from build123d import *

# Parameters (mm, degrees)
BOSS_EXTRUDE1_DEPTH = 4
SKETCH2_W           = 30
SKETCH2_H           = 22
BOSS_EXTRUDE2_DEPTH = 4
SKETCH3_W           = 30
SKETCH3_H           = 4
BOSS_EXTRUDE3_DEPTH = 18
CUT_EXTRUDE1_REACH  = 6
SKETCH4_R           = 2.25
CUT_EXTRUDE2_REACH  = 6
SKETCH5_W           = 12
SKETCH5_H           = 18


with BuildPart() as part:
    # Sketch1 → Boss-Extrude1 (new body)
    with BuildSketch(Plane(origin=(0, 0, 0), x_dir=(1, 0, 0), z_dir=(0, 1, 0))):
        with BuildLine():
            Line((-15, -14.5), (-9.788986692, -14.5))
            ThreePointArc((-9.788986692, -14.5), (-9, -10.35), (-8.211013308, -14.5))
            Line((-8.211013308, -14.5), (8.211013308, -14.5))
            ThreePointArc((8.211013308, -14.5), (9, -10.35), (9.788986692, -14.5))
            Line((9.788986692, -14.5), (15, -14.5))
            Line((15, -14.5), (15, 14.5))
            Line((15, 14.5), (-15, 14.5))
            Line((-15, 14.5), (-15, -14.5))
        make_face()
    extrude(amount=BOSS_EXTRUDE1_DEPTH)

    # Sketch2 → Boss-Extrude2 (add)
    with BuildSketch(Plane.XZ):
        with Locations((0, -3.5)):
            Rectangle(SKETCH2_W, SKETCH2_H)
    extrude(amount=BOSS_EXTRUDE2_DEPTH)

    # Sketch3 → Boss-Extrude3 (add)
    with BuildSketch(Plane(origin=(0, 0, -14.5), x_dir=(-1, 0, 0), z_dir=(0, 0, -1))):
        with Locations((0, 2)):
            Rectangle(SKETCH3_W, SKETCH3_H)
    extrude(amount=BOSS_EXTRUDE3_DEPTH)

    # Sketch4 → Cut-Extrude1 (cut, up to next)
    with BuildSketch(Plane(origin=(0, 0, 0), x_dir=(-1, 0, 0), z_dir=(0, 1, 0)), mode=Mode.PRIVATE) as cut_extrude1_sk1:
        with Locations((2, -27)):
            Circle(SKETCH4_R)
    cut_extrude1_tool1 = extrude(cut_extrude1_sk1.sketch, amount=CUT_EXTRUDE1_REACH, mode=Mode.PRIVATE) & part.part
    add(cut_extrude1_tool1.solids().sort_by_distance((-2, 0, -27))[0], mode=Mode.SUBTRACT)
    # Sketch4 → Cut-Extrude1 (cut, up to next)
    with BuildSketch(Plane(origin=(0, 0, 0), x_dir=(-1, 0, 0), z_dir=(0, 1, 0)), mode=Mode.PRIVATE) as cut_extrude1_sk2:
        with Locations((10, -23.5)):
            Circle(SKETCH4_R)
    cut_extrude1_tool2 = extrude(cut_extrude1_sk2.sketch, amount=CUT_EXTRUDE1_REACH, mode=Mode.PRIVATE) & part.part
    add(cut_extrude1_tool2.solids().sort_by_distance((-10, 0, -23.5))[0], mode=Mode.SUBTRACT)
    # Sketch4 → Cut-Extrude1 (cut, up to next)
    with BuildSketch(Plane(origin=(0, 0, 0), x_dir=(-1, 0, 0), z_dir=(0, 1, 0)), mode=Mode.PRIVATE) as cut_extrude1_sk3:
        with Locations((2, -20)):
            Circle(SKETCH4_R)
    cut_extrude1_tool3 = extrude(cut_extrude1_sk3.sketch, amount=CUT_EXTRUDE1_REACH, mode=Mode.PRIVATE) & part.part
    add(cut_extrude1_tool3.solids().sort_by_distance((-2, 0, -20))[0], mode=Mode.SUBTRACT)

    # Sketch5 → Cut-Extrude2 (cut, up to next)
    with BuildSketch(Plane(origin=(0, 0, 0), x_dir=(1, 0, 0), z_dir=(0, 1, 0)), mode=Mode.PRIVATE) as cut_extrude2_sk1:
        with Locations((9, 23.5)):
            Rectangle(SKETCH5_W, SKETCH5_H)
    cut_extrude2_tool1 = extrude(cut_extrude2_sk1.sketch, amount=CUT_EXTRUDE2_REACH, mode=Mode.PRIVATE) & part.part
    add(cut_extrude2_tool1.solids().sort_by_distance((9, 0, -23.5))[0], mode=Mode.SUBTRACT)


solid = part.part
Work out the finished part from the listing and answer in its coordinate system (mm). A direction names the side the tool comes from. Give positions to 0.01 mm unless a question says otherwise; leave off trailing zeros. Order: outer loops, then holes, each group sorted by start corner. A loop starts at its lowest first (then second) coordinate and runs counter-clockwise, first axis right, second up. Notation, with made-up numbers: (-18, 74) -> (-14, 74) arc R19 ccw to (-14, 107) -> close; hole circle Ø7 at (57, 87). An arc over 180 degrees is marked (long way). Answer as a JSON object with one key per item and string values. Group by question number.
1. Consider line 1 along X through (y, z) = (1.4, 12.5); line 2 along Z through (x, y) = (-2, 1.9); line 3 along X through (y, z) = (0.75, 11). Determine where each line is inside the solid, lowest interval first. Write a range as [from, to].
2. A tool of negligible diameter and unlimited length cuts with its end or side. For faces 1 (the flat face through (0, 0, 11)), 2 (the flat face through (-6, 0, -23)), 3 (the flat face through (3, 2, -23)), from which of +Z, -Z, +X, -X, +Y, -Y can it reach the whole face along a straight path? Write none if from no direction.
3. Section C-C on x = -2 is taken. Determine the outline of the cut face in (y, z).
4. Section A-A on z = 12.5 is taken. Determine the outline of the cut face in (x, y).
5. Section D-D on x = -9 is taken. Determine the outline of the cut face in (y, z).
6. Section B-B on y = 2.25 is taken. Determine the outline of the cut face in (x, z).
7. The mould has two halves that part along X. Classify faces 4 (the cylindrical face through (-1.512, 1.972, -29.196)), 5 (the flat face through (3, -1, -14.5)), 6 (the flat face through (15, 0, 0)): released by +X, released by -X, zero draft, split by the parting line, or undercut.
8. Flat-ended cylindrical pins translate along their axes: pin 1 Ø5.5 at (x, z) = (9, 12.5) entering from -Y; pin 2 Ø2.5 at (x, z) = (-10, -23.5) entering from +Y; pin 3 Ø1.2 at (x, y) = (3.5, -2.5) entering from +Z; pin 4 Ø2 at (y, z) = (2, -20) entering from +X. Find the tip coordinate at first contact, or state that the pin passes through.
Result sheet:
{
 "1": {"line 1": "x = [-15, -11.15], [-6.85, 6.85], [11.15, 15]", "line 2": "z = [-32.5, -29.25], [-24.75, -22.25], [-17.75, 14.5]", "line 3": "x = [-15, -10.54], [-7.46, 7.46], [10.54, 15]"},
 "2": {"face 1": "+Z, +X, -X, -Y", "face 2": "-Z, +X, -X, -Y", "face 3": "-Z, +X, +Y, -Y"},
 "3": {"outline": "(-4, -14.5) -> (0, -14.5) -> (0, -17.75) -> (4, -17.75) -> (4, 14.5) -> (0, 14.5) -> (0, 7.5) -> (-4, 7.5) -> close; (0, -32.5) -> (4, -32.5) -> (4, -29.25) -> (0, -29.25) -> close; (0, -24.75) -> (4, -24.75) -> (4, -22.25) -> (0, -22.25) -> close"},
 "4": {"outline": "(-15, 0) -> (-11.15, 0) -> (-11.15, 4) -> (-15, 4) -> close; (-6.85, 0) -> (6.85, 0) -> (6.85, 4) -> (-6.85, 4) -> close; (11.15, 0) -> (15, 0) -> (15, 4) -> (11.15, 4) -> close"},
 "5": {"outline": "(-4, -14.5) -> (0, -14.5) -> (0, -21.48) -> (4, -21.48) -> (4, 10.35) -> (0, 10.35) -> (0, 7.5) -> (-4, 7.5) -> close; (0, -32.5) -> (4, -32.5) -> (4, -25.52) -> (0, -25.52) -> close"},
 "6": {"outline": "(-15, -32.5) -> (3, -32.5) -> (3, -14.5) -> (15, -14.5) -> (15, 14.5) -> (9.79, 14.5) arc R2.15 cw (long way) to (8.21, 14.5) -> (-8.21, 14.5) arc R2.15 cw (long way) to (-9.79, 14.5) -> (-15, 14.5) -> close; hole circle Ø4.5 at (-10, -23.5); hole circle Ø4.5 at (-2, -27); hole circle Ø4.5 at (-2, -20)"},
 "7": {"face 4": "undercut", "face 5": "zero draft", "face 6": "released by +X"},
 "8": {"pin 1": "stops at y = 0", "pin 2": "passes through", "pin 3": "stops at z = 7.5", "pin 4": "stops at x = 3"}
}
